Source: CAD feature listing. Evaluate the final solid. Frame: model axes, mm. A direction names the side the tool comes from. Round coordinates to 2 decimals unless told otherwise and drop trailing zeros. Write each loop counter-clockwise with the first axis right and the second up, starting at its lowest first coordinate (ties: lowest second). Pieces come first, ordered by that corner, then holes. Notation, with made-up numbers: (37, 67.25) -> (62, 67.25) arc R7 ccw to (62, 76.25) -> close; hole circle Ø10 at (-21.75, 74). An arc over 180 degrees is marked (long way). Put each result on its own line as item: value.
```python
from build123d import *

# Parameters (mm, degrees)
SKETCH_1_R          = 11
EXTRUDE_1_DEPTH     = 3.5
SKETCH_2_R          = 4
CUT_EXTRUDE_1_DEPTH = 8
SKETCH_3_R          = 9.6
SKETCH_3_R_2        = 6.05
CUT_EXTRUDE_2_DEPTH = 0.5


with BuildPart() as part:
    # 草圖1 → 填料-伸長1 (new body, symmetric)
    with BuildSketch(Plane.XY):
        Circle(SKETCH_1_R)
    extrude(amount=EXTRUDE_1_DEPTH, both=True)

    # 草圖2 → 除料-伸長1 (cut, through all)
    with BuildSketch(Plane.XY.offset(3.5)):
        Circle(SKETCH_2_R)
    extrude(amount=-CUT_EXTRUDE_1_DEPTH, mode=Mode.SUBTRACT)

    # 草圖3 → 除料-伸長2 (cut)
    with BuildSketch(Plane.XY.offset(3.5)):
        Circle(SKETCH_3_R)
        Circle(SKETCH_3_R_2, mode=Mode.SUBTRACT)
    cut_extrude_2 = extrude(amount=-CUT_EXTRUDE_2_DEPTH, mode=Mode.SUBTRACT)

    # 鏡射1: 除料-伸長2 across plane
    add(cut_extrude_2.mirror(Plane.XY), mode=Mode.SUBTRACT)


solid = part.part
```
Q1. Pin query (flat end, axial travel): pin 1 (3 mm diameter, centred on x = 5.5, z = -2, fed in from +Y); pin 2 (3 mm diameter, centred on x = -5.5, z = 0, fed in from -Y); pin 3 (1.5 mm diameter, centred on x = -8.5, z = 2.5, fed in from +Y); pin 4 (1.5 mm diameter, centred on x = -2.5, y = -1, fed in from -Z). Return the tip coordinate at first contact, or that it passes through.
Ans:
pin 1: stops at y = 10.25
pin 2: stops at y = -10.25
pin 3: stops at y = 7.81
pin 4: passes through
Q2. Cut plane A-A on y = 0. Output: boundary loops of the cut face in (x, z), and give its area (3 significant figures).
Ans:
outline: (-11, -3.5) -> (-9.6, -3.5) -> (-9.6, -3) -> (-6.05, -3) -> (-6.05, -3.5) -> (-4, -3.5) -> (-4, 3.5) -> (-6.05, 3.5) -> (-6.05, 3) -> (-9.6, 3) -> (-9.6, 3.5) -> (-11, 3.5) -> close; (4, -3.5) -> (6.05, -3.5) -> (6.05, -3) -> (9.6, -3) -> (9.6, -3.5) -> (11, -3.5) -> (11, 3.5) -> (9.6, 3.5) -> (9.6, 3) -> (6.05, 3) -> (6.05, 3.5) -> (4, 3.5) -> close
area: 90.9 mm^2
Q3. Draft query along X for faces 1 (the cylindrical face through (-2.38, -10.74, 0.05)), 2 (the cylindrical face through (5.161, 8.095, -3.254)), 3 (the flat face through (1, 10, 3.5)). Return one class per face: +X half, -X half, draft (parallel to the pull), parting line (faces both ways), or undercut.
Ans:
face 1: parting line
face 2: undercut
face 3: draft
Q4. Reachability of faces 4 (the cylindrical face through (5.589, -2.317, -3.254)), 5 (the cylindrical face through (5.589, -2.317, 3.254)), 6 (the cylindrical face through (-0.867, -3.905, 0.049)) from +Z, -Z, +X, -X, +Y, -Y: full face, straight path, thin tool, end or side. Return the list, or none.
Ans:
face 4: -Z
face 5: +Z
face 6: +Z, -Z
Q5. Cut plane D-D on x = 8.25. Output: boundary loops of the cut face in (y, z), and give its area (3 significant figures).
Ans:
outline: (-7.28, -3.5) -> (-4.91, -3.5) -> (-4.91, -3) -> (4.91, -3) -> (4.91, -3.5) -> (7.28, -3.5) -> (7.28, 3.5) -> (4.91, 3.5) -> (4.91, 3) -> (-4.91, 3) -> (-4.91, 3.5) -> (-7.28, 3.5) -> close
area: 92.0 mm^2
Q6. Cut plane C-C on z = -1. Output: boundary loops of the cut face in (x, y), and give its area (3 significant figures).
Ans:
outline: circle Ø22 at (0, 0); hole circle Ø8 at (0, 0)
area: 330 mm^2
Q7. Material intervals for line 1 (Y direction, x = 0, z = 3.25); line 2 (Y direction, x = 0, z = -1.5); line 3 (Z direction, x = -3.25, y = 7.75), sorted ascending. Write a range as [from, to].
Ans:
line 1: y = [-11, -9.6], [-6.05, -4], [4, 6.05], [9.6, 11]
line 2: y = [-11, -4], [4, 11]
line 3: z = [-3, 3]
